```python
from build123d import *

# Parameters (mm, degrees)
BOSS_EXTRUDE1_DEPTH = 304.8
SKETCH7_W           = 25.4
SKETCH7_H           = 165.1
CUT_EXTRUDE1_DEPTH  = 254
SKETCH3_R           = 2.5
CUT_EXTRUDE2_DEPTH  = 254
SKETCH8_R           = 2.5
CUT_EXTRUDE4_DEPTH  = 254


with BuildPart() as part:
    # Sketch2 → Boss-Extrude1 (new, symmetric)
    with BuildSketch(Plane.XY):
        with BuildLine():
            Line((-12.7, -12.7), (12.7, -12.7))
            Line((12.7, -12.7), (12.7, 12.7))
            Line((12.7, 12.7), (11.1125, 12.7))
            ThreePointArc((11.1125, 12.7), (9.989967985, 12.235032015), (9.525, 11.1125))
            Line((9.525, 11.1125), (9.525, -6.35))
            ThreePointArc((9.525, -6.35), (8.59506403, -8.59506403), (6.35, -9.525))
            Line((6.35, -9.525), (-11.1125, -9.525))
            ThreePointArc((-11.1125, -9.525), (-12.235032015, -9.989967985), (-12.7, -11.1125))
            Line((-12.7, -11.1125), (-12.7, -12.7))
        make_face()
    extrude(amount=BOSS_EXTRUDE1_DEPTH, both=True)

    # Sketch7 → Cut-Extrude1 (cut)
    with BuildSketch(Plane.XZ.offset(12.7)):
        with Locations((0, 222.25)):
            Rectangle(SKETCH7_W, SKETCH7_H)
    extrude(amount=-CUT_EXTRUDE1_DEPTH, mode=Mode.SUBTRACT)

    # Sketch3 → Cut-Extrude2 (cut)
    with BuildSketch(Plane(origin=(0, 0, 0), x_dir=(1, 0, 0), z_dir=(0, 1, 0))):
        with Locations(Location((-6.35, 292.1, 0), (0, 0, 270))):
            Circle(SKETCH3_R)
        with Locations(Location((0, 298.45, 0), (0, 0, 270))):
            Circle(SKETCH3_R)
        with Locations(Location((0, 273.05, 0), (0, 0, 270))):
            Circle(SKETCH3_R)
        with Locations(Location((0, 234.95, 0), (0, 0, 270))):
            Circle(SKETCH3_R)
        with Locations(Location((0, 196.85, 0), (0, 0, 270))):
            Circle(SKETCH3_R)
        with Locations(Location((0, 158.75, 0), (0, 0, 270))):
            Circle(SKETCH3_R)
        with Locations(Location((0, 120.65, 0), (0, 0, 270))):
            Circle(SKETCH3_R)
        with Locations(Location((0, 82.55, 0), (0, 0, 270))):
            Circle(SKETCH3_R)
        with Locations(Location((0, 44.45, 0), (0, 0, 270))):
            Circle(SKETCH3_R)
        with Locations(Location((0, 6.35, 0), (0, 0, 270))):
            Circle(SKETCH3_R)
        with Locations(Location((0, -31.75, 0), (0, 0, 270))):
            Circle(SKETCH3_R)
        with Locations(Location((0, -69.85, 0), (0, 0, 270))):
            Circle(SKETCH3_R)
        with Locations(Location((0, -107.95, 0), (0, 0, 270))):
            Circle(SKETCH3_R)
        with Locations(Location((0, -133.35, 0), (0, 0, 270))):
            Circle(SKETCH3_R)
        with Locations(Location((-6.35, -127, 0), (0, 0, 270))):
            Circle(SKETCH3_R)
    extrude(amount=-CUT_EXTRUDE2_DEPTH, mode=Mode.SUBTRACT)

    # Sketch8 → Cut-Extrude4 (cut)
    with BuildSketch(Plane(origin=(12.7, 0, -12.7), x_dir=(0, 0, 1), z_dir=(-1, 0, 0))):
        with Locations(Location((136.525, 6.35, 0), (0, 0, 90))):
            Circle(SKETCH8_R)
        with Locations(Location((142.875, 0, 0), (0, 0, 90))):
            Circle(SKETCH8_R)
        with Locations(Location((120.65, -3.175, 0), (0, 0, 90))):
            Circle(SKETCH8_R)
        with Locations(Location((82.55, -3.175, 0), (0, 0, 90))):
            Circle(SKETCH8_R)
        with Locations(Location((44.45, -3.175, 0), (0, 0, 90))):
            Circle(SKETCH8_R)
        with Locations(Location((6.35, -3.175, 0), (0, 0, 90))):
            Circle(SKETCH8_R)
        with Locations(Location((-31.75, -3.175, 0), (0, 0, 90))):
            Circle(SKETCH8_R)
        with Locations(Location((-69.85, -3.175, 0), (0, 0, 90))):
            Circle(SKETCH8_R)
        with Locations(Location((-107.95, -3.175, 0), (0, 0, 90))):
            Circle(SKETCH8_R)
        with Locations(Location((-146.05, -3.175, 0), (0, 0, 90))):
            Circle(SKETCH8_R)
        with Locations(Location((-184.15, -3.175, 0), (0, 0, 90))):
            Circle(SKETCH8_R)
        with Locations(Location((-222.25, -3.175, 0), (0, 0, 90))):
            Circle(SKETCH8_R)
        with Locations(Location((-260.35, -3.175, 0), (0, 0, 90))):
            Circle(SKETCH8_R)
        with Locations(Location((-282.575, 0, 0), (0, 0, 90))):
            Circle(SKETCH8_R)
        with Locations(Location((-276.225, 6.35, 0), (0, 0, 90))):
            Circle(SKETCH8_R)
    extrude(amount=CUT_EXTRUDE4_DEPTH, mode=Mode.SUBTRACT)


solid = part.part
```
Work out the finished part from the listing and answer in its coordinate system (mm). A direction names the side the tool comes from. Give positions to 0.01 mm unless a question says otherwise; leave off trailing zeros. One line per item, written item: value. Start each with the question number.
1. Each of these flat-tipped pins is pushed along its axis until it touches: P1, Ø1.5, axis at y = 0, z = -222.5, coming from the -X side (3 decimals); P2, Ø8, axis at y = -3.175, z = -234.95, coming from the -X side; P3, Ø6, axis at x = 0, z = -298.45, coming from the +Y side (3 decimals). Where does it stop, or does it pass through?
2. Which of the six approach directions +Z, -Z, +X, -X, +Y, -Y give full straight-line access (tool end or side, diameter ignored) to faces 1 (the face through (0, -12.7, -79)), 2 (the face through (9.525, 3, -79))?
3. Find the intervals of material crossed by probe 1 along Z at (x, y) = (10.5, 8.5); probe 2 along Y at (x, z) = (-9, -58) (3 decimals); probe 3 along X at (y, z) = (4, 42.5) (3 decimals), in increasing order.
Reported:
1. P1: stops at x = 9.525
1. P2: stops at x = 9.42
1. P3: stops at y = -9.525
2. face 1: +Z, -Z, +X, -X, -Y
2. face 2: +Z, -Z, -X, +Y
3. probe 1: z = -304.8 to -290.2, -287.65 to 122.55, 125.1 to 139.7
3. probe 2: y = -12.7 to -9.525
3. probe 3: x = 9.525 to 12.7
